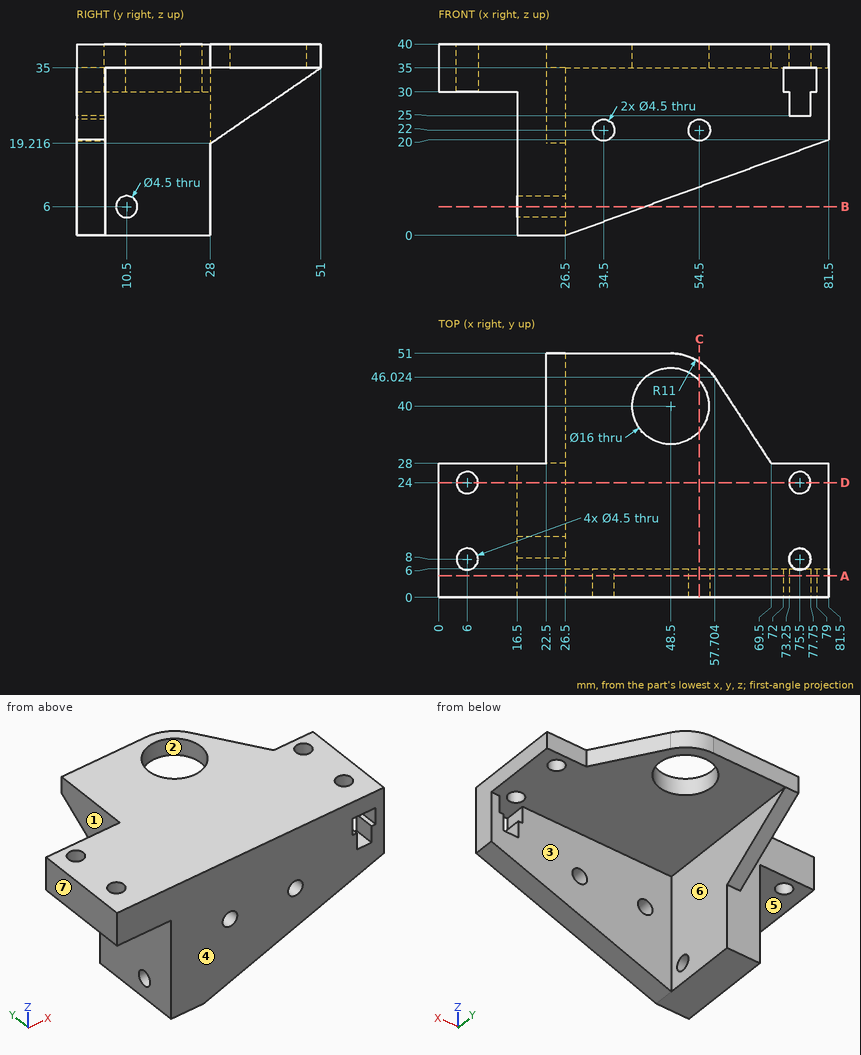
Answer from the drawing. Dimensions are ordinates in mm from the lowest x, y and z of the part. A direction names the side the tool comes from. Round coordinates to 2 decimals unless told otherwise and drop trailing zeros. Loops run counter-clockwise (first coordinate to the right, second up) from the corner with the lowest first, then second, coordinate; pieces in that order, holes last.
1) A cutting plane is placed at C-C on x = 54.5. Determine the outline of the cut face in (y, z), plus the area to 3 significant figures.
Outcome:
outline: (0, 10.18) - (6, 10.18) - (6, 19.75) - (0, 19.75) - close; (0, 24.25) - (6, 24.25) - (6, 35) - (34.71, 35) - (34.71, 40) - (0, 40) - close; (45.29, 35) - (49.22, 35) - (49.22, 40) - (45.29, 40) - close
area: 315 mm2
2) For the marked faces 5, 6 and 7, determine the directions among +Z, -Z, +X, -X, +Y, -Y from which every point of the face is accessible in a straight line to the end or side of a thin tool.
Outcome:
face 5: -Z, -X, +Y, -Y
face 6: -Z, +X, +Y
face 7: +Z, -Z, -X, +Y, -Y
3) Consider line 1 (Y direction, x = 75.5, z = 37.1); line 2 (X direction, y = 23.5, z = 36.5); line 3 (Y direction, x = 48.5, z = 37.5). Determine where each line is inside the solid, lowest interval first.
Outcome:
line 1: y = 0 to 5.75, 10.25 to 21.75, 26.25 to 28
line 2: x = 0 to 3.81, 8.19 to 73.31, 77.69 to 81.5
line 3: y = 0 to 32, 48 to 51
4) A cutting plane is placed at B-B on z = 6. Determine the outline of the cut face in (x, y), plus the area to 3 significant figures.
Outcome:
outline: (16.5, 0) - (43, 0) - (43, 6) - (26.5, 6) - (26.5, 8.25) - (16.5, 8.25) - close; (16.5, 12.75) - (26.5, 12.75) - (26.5, 28) - (16.5, 28) - close
area: 334 mm2
5) A cutting plane is placed at A-A on y = 4.5. Determine the outline of the cut face in (x, z), plus the area to 3 significant figures.
Outcome:
outline: (0, 30) - (16.5, 30) - (16.5, 0) - (26.5, 0) - (81.5, 20) - (81.5, 40) - (0, 40) - close; hole circle Ø4.5 at (34.5, 22); hole circle Ø4.5 at (54.5, 22); hole (72, 30) - (73.25, 30) - (73.25, 25) - (77.75, 25) - (77.75, 30) - (79, 30) - (79, 35) - (72, 35) - close
area: 2,130 mm2
6) Given P1, Ø4, axis at y = 15.5, z = 12, coming from the +X side; P2, Ø12, axis at y = 23.5, z = 14.5, coming from the -X side; P3, Ø4, axis at x = 19, y = 37.5, coming from the -Z side; P4, Ø8, axis at x = 7, y = 10, coming from the -Z side, each flat-ended and moving along its own axis, determine where each tip first touches the part or whether it passes through.
Outcome:
P1: stops at x = 26.5
P2: stops at x = 16.5
P3: passes through
P4: stops at z = 30
7) For a pull along Y with two mould halves and no side action, classify the marked faces 1, 2, 3 and 4 as released by +Y, released by -Y, zero draft, split by the parting line, or undercut.
Outcome:
face 1: zero draft
face 2: undercut
face 3: released by +Y
face 4: released by -Y
8) A cutting plane is placed at D-D on y = 24. Determine the outline of the cut face in (x, z).
Outcome:
outline: (0, 30) - (3.75, 30) - (3.75, 40) - (0, 40) - close; (8.25, 30) - (16.5, 30) - (16.5, 0) - (26.5, 0) - (26.5, 35) - (73.25, 35) - (73.25, 40) - (8.25, 40) - close; (77.75, 35) - (81.5, 35) - (81.5, 40) - (77.75, 40) - close
